Build history of the part. All positions in model axes, mm. Face numbers are marked on the shaded views. A direction names the side the tool comes from. Coordinates: 2 decimals unless noted, no trailing zeros. Loops run counter-clockwise (first coordinate to the right, second up) from the corner with the lowest first, then second, coordinate; pieces in that order, holes last.
Item 1: Drill centre lines: line 1 along Y through (x, z) = (5.5, 9.5); line 2 along Y through (x, z) = (112, 6); line 3 along X through (y, z) = (26, 7). Where is each one in solid material? Low to high.
Item 2: 3-axis set-ups, long thin cutter, end or side, ignore diameter. For the marked faces 5, 6 and 7: which of +Z, -Z, +X, -X, +Y, -Y reach the whole face in a straight line?
Item 3: Cut at B-B (x = 100). List the corners of the cut face in (y, z), and give its area (3 significant figures).
Item 4: Mould opens along X. For the marked faces 1, 2, 3 and 4 say: released by +X, released by -X, zero draft, split by the parting line, or undercut.
Item 5: Flat gauge pins, fed straight in: pin 1 (12 mm diameter, centred on x = 57, y = 47.5, fed in from +Z); pin 2 (2.5 mm diameter, centred on x = 104.5, z = 11, fed in from -Y); pin 3 (1.2 mm diameter, centred on x = 65.5, z = -7.5, fed in from +Y). Where does each tip first touch, or does it go through?
Item 6: Cut at C-C (z = -25). List the corners of the cut face in (x, y), and give its area (3 significant figures).
Item 7: Cut at D-D (x = 26). List the corners of the cut face in (y, z), and give its area (3 significant figures).
Item 8: Cut at A-A (y = 42.4). List the corners of the cut face in (x, z).
from build123d import *

# Parameters (mm, degrees)
SKETCH1_W               = 120
SKETCH1_H               = 45.4
BOSS_EXTRUDE1_DEPTH     = 12.5
SKETCH2_W               = 5
SKETCH2_H               = 45.4
BOSS_EXTRUDE2_DEPTH     = 10
CUT_EXTRUDE1_DEPTH      = 7.5
CUT_EXTRUDE1_DEPTH_BACK = 129.908533465
SKETCH3_W               = 78
SKETCH3_H               = 12.2
BOSS_EXTRUDE3_START     = -12.5
SKETCH4_W               = 42
SKETCH4_H               = 41
BOSS_EXTRUDE3_DEPTH     = 12.5
SKETCH5_R               = 15
SKETCH5_R_2             = 1.7
CUT_EXTRUDE2_DEPTH      = 138.38722648
SKETCH7_W               = 30
SKETCH7_H               = 8
BOSS_EXTRUDE4_DEPTH     = 44.5
SKETCH8_R               = 1.65
CUT_EXTRUDE4_DEPTH      = 148.030609058
FILLET1_SIZE            = 15
FILLET1_SIZE_2          = 6
SKETCH9_R               = 2.599999999
SKETCH9_R_2             = 12.000000007
CUT_EXTRUDE5_DEPTH      = 10
SKETCH10_R              = 3.5
CUT_EXTRUDE6_DEPTH      = 10.5
SKETCH12_R              = 3.5
CUT_EXTRUDE7_DEPTH      = 7.5
SKETCH6_W               = 105.644224039
SKETCH6_H               = 30.4
CUT_EXTRUDE3_DEPTH      = 10.5
CHAMFER1_SIZE           = 5
CHAMFER1_SIZE2          = 13.737387097
SKETCH13_W              = 14
SKETCH13_H              = 32.158687744
CUT_EXTRUDE8_DEPTH      = 10
SKETCH16_W              = 22.5
SKETCH16_H              = 11
CUT_EXTRUDE9_DEPTH      = 2
SKETCH18_W              = 3
SKETCH18_H              = 10.169703164
BOSS_EXTRUDE7_DEPTH     = 9.5
CUT_EXTRUDE10_REACH     = 144.298
SKETCH19_W              = 1.5
SKETCH19_H              = 14
SKETCH20_W              = 20
SKETCH20_H              = 5
CUT_EXTRUDE11_DEPTH     = 11
SKETCH21_R              = 1.5
CUT_EXTRUDE12_DEPTH     = 7
CHAMFER3_SIZE           = 1.5
FILLET3_R               = 5
CUT_EXTRUDE16_REACH     = 144.298
SKETCH24_W              = 5
SKETCH24_H              = 9
BOSS_EXTRUDE8_DEPTH     = 12.2
FILLET4_R               = 1
SKETCH15_R              = 2.75
BOSS_EXTRUDE9_DEPTH     = 2
CHAMFER4_SIZE           = 2
CHAMFER5_DEPTH          = 8


with BuildPart() as part:
    # Sketch1 → Boss-Extrude1 (new body)
    with BuildSketch(Plane.XY):
        with Locations((60, 22.7)):
            Rectangle(SKETCH1_W, SKETCH1_H)
    extrude(amount=BOSS_EXTRUDE1_DEPTH)

    # Sketch2 → Boss-Extrude2 (add)
    with BuildSketch(Plane(origin=(0, 0, 0), x_dir=(-1, 0, 0), z_dir=(0, 0, -1))):
        with Locations((-117.5, 22.7)):
            Rectangle(SKETCH2_W, SKETCH2_H)
    extrude(amount=BOSS_EXTRUDE2_DEPTH)

    # Sketch3 → Cut-Extrude1 (cut, two sides: drawn at the far end of the back side and taken through both)
    with BuildSketch(Plane.XY.offset(-CUT_EXTRUDE1_DEPTH_BACK)):
        with Locations((81, 22.8)):
            Rectangle(SKETCH3_W, SKETCH3_H)
    extrude(amount=CUT_EXTRUDE1_DEPTH + CUT_EXTRUDE1_DEPTH_BACK, mode=Mode.SUBTRACT)

    # Sketch4 → Boss-Extrude3 (add)
    with BuildSketch(Plane(origin=(0, 0, 0), x_dir=(-1, 0, 0), z_dir=(0, 0, -1)).offset(BOSS_EXTRUDE3_START)):
        with Locations((-21, 42.5)):
            Rectangle(SKETCH4_W, SKETCH4_H)
    extrude(amount=BOSS_EXTRUDE3_DEPTH)

    # Sketch5 → Cut-Extrude2 (cut, through all)
    with BuildSketch(Plane.XY.offset(12.5)):
        with Locations((21, 42.4)):
            Circle(SKETCH5_R)
        with Locations((5.5, 57.9)):
            Circle(SKETCH5_R_2)
        with Locations((36.5, 57.9)):
            Circle(SKETCH5_R_2)
        with Locations((36.5, 26.9)):
            Circle(SKETCH5_R_2)
        with Locations((5.5, 26.9)):
            Circle(SKETCH5_R_2)
    extrude(amount=-CUT_EXTRUDE2_DEPTH, mode=Mode.SUBTRACT)

    # Sketch7 → Boss-Extrude4 (add)
    with BuildSketch(Plane(origin=(0, 0, 0), x_dir=(-1, 0, 0), z_dir=(0, 0, -1))):
        with Locations((-65.5, 4)):
            Rectangle(SKETCH7_W, SKETCH7_H)
    extrude(amount=BOSS_EXTRUDE4_DEPTH)

    # Sketch8 → Cut-Extrude4 (cut, through all)
    with BuildSketch(Plane.XY.offset(12.5)):
        with Locations((91.5, 32.7)):
            Circle(SKETCH8_R)
        with Locations((111.5, 32.7)):
            Circle(SKETCH8_R)
        with Locations((111.5, 12.7)):
            Circle(SKETCH8_R)
        with Locations((91.5, 12.7)):
            Circle(SKETCH8_R)
    extrude(amount=-CUT_EXTRUDE4_DEPTH, mode=Mode.SUBTRACT)

    # Fillet1
    # a fillet whose section is not a circle: 15, 6 mm, written as the material it takes off along each edge
    with BuildSketch(Plane(origin=(50.5, -37.5, -44.5), x_dir=(1, 0, 0), z_dir=(0, 1, 0))) as fillet1_piece_1:
        with BuildLine():
            Bezier((FILLET1_SIZE, 0), (0, 0), (0, -FILLET1_SIZE_2), weights=[1, 0.428571429, 1])
            Line((0, -FILLET1_SIZE_2), (0, 0))
            Line((0, 0), (FILLET1_SIZE, 0))
        make_face()
    extrude(amount=83, mode=Mode.SUBTRACT)
    with BuildSketch(Plane(origin=(80.5, 45.5, -44.5), x_dir=(0, 0, 1), z_dir=(0, -1, 0))) as fillet1_piece_2:
        with BuildLine():
            Bezier((FILLET1_SIZE_2, 0), (0, 0), (0, FILLET1_SIZE), weights=[1, 0.428571429, 1])
            Line((0, FILLET1_SIZE), (0, 0))
            Line((0, 0), (FILLET1_SIZE_2, 0))
        make_face()
    extrude(amount=83, mode=Mode.SUBTRACT)

    # Sketch9 → Cut-Extrude5 (cut)
    with BuildSketch(Plane(origin=(0, 8, 0), x_dir=(1, 0, 0), z_dir=(0, 1, 0))):
        with Locations(Location((54.15539193, 34.815048574, 0), (0, 0, 180))):
            Circle(SKETCH9_R)
        with Locations(Location((65.469100429, 39.501340075, 0), (0, 0, 180))):
            Circle(SKETCH9_R)
        with Locations(Location((76.782808928, 34.815048574, 0), (0, 0, 180))):
            Circle(SKETCH9_R)
        with Locations(Location((65.469100429, 23.501340075, 0), (0, 0, 180))):
            Circle(SKETCH9_R_2)
    extrude(amount=-CUT_EXTRUDE5_DEPTH, mode=Mode.SUBTRACT)

    # Sketch10 → Cut-Extrude6 (cut)
    with BuildSketch(Plane.XY.offset(12.5)):
        with Locations((91.5, 32.7)):
            Circle(SKETCH10_R)
        with Locations((111.5, 32.7)):
            Circle(SKETCH10_R)
        with Locations((111.5, 12.7)):
            Circle(SKETCH10_R)
        with Locations((91.5, 12.7)):
            Circle(SKETCH10_R)
    extrude(amount=-CUT_EXTRUDE6_DEPTH, mode=Mode.SUBTRACT)

    # Sketch12 → Cut-Extrude7 (cut)
    with BuildSketch(Plane.XY.offset(12.5)):
        with Locations((36.5, 57.9)):
            Circle(SKETCH12_R)
        with Locations((5.5, 57.9)):
            Circle(SKETCH12_R)
        with Locations((5.5, 26.9)):
            Circle(SKETCH12_R)
        with Locations((36.5, 26.9)):
            Circle(SKETCH12_R)
    extrude(amount=-CUT_EXTRUDE7_DEPTH, mode=Mode.SUBTRACT)

    # Sketch6 → Cut-Extrude3 (cut)
    with BuildSketch(Plane.XY.offset(12.5)):
        with Locations((73.822112019, 47.8)):
            Rectangle(SKETCH6_W, SKETCH6_H)
    extrude(amount=-CUT_EXTRUDE3_DEPTH, mode=Mode.SUBTRACT)

    # Chamfer1
    chamfer1_edges = [part.edges().sort_by_distance(p)[0] for p in [
        (80.5, 4, 0),
    ]]
    chamfer1_side = [part.faces().sort_by_distance(p)[0] for p in [
        (40.688741063, 22.8, 0),
    ]]
    chamfer(chamfer1_edges, length=CHAMFER1_SIZE, length2=CHAMFER1_SIZE2, reference=chamfer1_side[0])

    # Sketch13 → Cut-Extrude8 (cut)
    with BuildSketch(Plane(origin=(0, 8, 0), x_dir=(1, 0, 0), z_dir=(0, 1, 0))):
        with Locations((65.469100429, 39.501340075)):
            Rectangle(SKETCH13_W, SKETCH13_H)
    extrude(amount=-CUT_EXTRUDE8_DEPTH, mode=Mode.SUBTRACT)

    # Sketch16 → Cut-Extrude9 (cut)
    with BuildSketch(Plane(origin=(120, 0, 0), x_dir=(0, 0, -1), z_dir=(1, 0, 0))):
        with Locations((-1.25, 5.5)):
            Rectangle(SKETCH16_W, SKETCH16_H)
    extrude(amount=-CUT_EXTRUDE9_DEPTH, mode=Mode.SUBTRACT)

    # Sketch18 → Boss-Extrude7 (add)
    with BuildSketch(Plane(origin=(0, 0, -10), x_dir=(-1, 0, 0), z_dir=(0, 0, -1))):
        with Locations((-116.5, 5.084851582)):
            Rectangle(SKETCH18_W, SKETCH18_H)
    extrude(amount=BOSS_EXTRUDE7_DEPTH)

    # Cut-Extrude10: up to this face of the body (flat: up to its plane)
    cut_extrude10_end = Plane(part.part.faces().sort_by_distance((119, 11, 1.25))[0])
    # Sketch19 → Cut-Extrude10 (cut, up to the picked face)
    with BuildSketch(Plane.XZ, mode=Mode.PRIVATE) as cut_extrude10_sk1:
        with Locations((117.25, -7)):
            Rectangle(SKETCH19_W, SKETCH19_H)
    cut_extrude10_tool1 = split(extrude(cut_extrude10_sk1.sketch, amount=-CUT_EXTRUDE10_REACH, mode=Mode.PRIVATE), bisect_by=cut_extrude10_end, keep=Keep.BOTH, mode=Mode.PRIVATE)
    add(cut_extrude10_tool1.solids().sort_by(Axis((117.25, 0, -7), (0, 1, 0)))[0], mode=Mode.SUBTRACT)

    # Sketch20 → Cut-Extrude11 (cut)
    with BuildSketch(Plane.XZ):
        with Locations((108, 10)):
            Rectangle(SKETCH20_W, SKETCH20_H)
    extrude(amount=-CUT_EXTRUDE11_DEPTH, mode=Mode.SUBTRACT)

    # Sketch21 → Cut-Extrude12 (cut)
    with BuildSketch(Plane(origin=(118, 0, 0), x_dir=(0, 0, -1), z_dir=(1, 0, 0))):
        with Locations((-2.485, 5)):
            Circle(SKETCH21_R)
        with Locations((16.565, 5)):
            Circle(SKETCH21_R)
    extrude(amount=-CUT_EXTRUDE12_DEPTH, mode=Mode.SUBTRACT)

    # Chamfer3
    chamfer3_edges = [part.edges().sort_by_distance(p)[0] for p in [
        (116.5, 5.084851582, -14),
        (116.5, 5.5, 0),
    ]]
    chamfer(chamfer3_edges, length=CHAMFER3_SIZE - 0.0001)  # a hair under: the kernel refuses the full size

    # Fillet3
    fillet3_edges = [part.edges().sort_by_distance(p)[0] for p in [
        (98, 11, 10),
    ]]
    fillet(fillet3_edges, radius=FILLET3_R)

    # Cut-Extrude16: up to this face of the body (flat: up to its plane)
    cut_extrude16_end = Plane(part.part.faces().sort_by_distance((42, 22.8, 3.75))[0])
    # Sketch23 → Cut-Extrude16 (cut, up to the picked face)
    with BuildSketch(Plane(origin=(120, 0, 0), x_dir=(0, 0, -1), z_dir=(1, 0, 0)), mode=Mode.PRIVATE) as cut_extrude16_sk1:
        Polygon((-6.5, 28.9), (-7.5, 28.9), (-7.5, 29.3), align=None)
    cut_extrude16_tool1 = split(extrude(cut_extrude16_sk1.sketch, amount=-CUT_EXTRUDE16_REACH, mode=Mode.PRIVATE), bisect_by=cut_extrude16_end, keep=Keep.BOTH, mode=Mode.PRIVATE)
    # Sketch23 → Cut-Extrude16 (cut, up to the picked face)
    with BuildSketch(Plane(origin=(120, 0, 0), x_dir=(0, 0, -1), z_dir=(1, 0, 0)), mode=Mode.PRIVATE) as cut_extrude16_sk2:
        Polygon((-7.5, 16.7), (-7.5, 16.3), (-6.5, 16.7), align=None)
    cut_extrude16_tool2 = split(extrude(cut_extrude16_sk2.sketch, amount=-CUT_EXTRUDE16_REACH, mode=Mode.PRIVATE), bisect_by=cut_extrude16_end, keep=Keep.BOTH, mode=Mode.PRIVATE)
    add(cut_extrude16_tool1.solids().sort_by(Axis((120, 29.033333, 7.166667), (-1, 0, 0)))[0], mode=Mode.SUBTRACT)
    add(cut_extrude16_tool2.solids().sort_by(Axis((120, 16.566667, 7.166667), (-1, 0, 0)))[0], mode=Mode.SUBTRACT)

    # Sketch24 → Boss-Extrude8 (add)
    with BuildSketch(Plane(origin=(0, 16.7, 0), x_dir=(1, 0, 0), z_dir=(0, 1, 0))):
        with Locations((117.5, 5.5)):
            Rectangle(SKETCH24_W, SKETCH24_H)
    extrude(amount=BOSS_EXTRUDE8_DEPTH)

    # Fillet4
    fillet4_edges = [part.edges().sort_by_distance(p)[0] for p in [
        (117.5, 28.9, -1),
        (117.5, 16.7, -1),
    ]]
    fillet(fillet4_edges, radius=FILLET4_R)

    # Sketch15 → Boss-Extrude9 (add)
    with BuildSketch(Plane(origin=(0, 8, 0), x_dir=(1, 0, 0), z_dir=(0, 1, 0))):
        with Locations((65.469100428, 7.501340074)):
            Circle(SKETCH15_R)
    extrude(amount=BOSS_EXTRUDE9_DEPTH)

    # Chamfer4
    chamfer4_edges = [part.edges().sort_by_distance(p)[0] for p in [
        (62.719100428, 10, -7.501340074),
    ]]
    chamfer(chamfer4_edges, length=CHAMFER4_SIZE - 0.0001)  # a hair under: the kernel refuses the full size

    # Chamfer5: read off the stored shape, not the designer's step
    # Chamfer5 outline → Chamfer5 (add)
    with BuildSketch(Plane(origin=(0, 0, 0), x_dir=(1, 0, 0), z_dir=(0, 1, 0))):
        with BuildLine():
            add(Edge.make_bspline(
                [(50.541922163, 38.782180687), (50.5, 38.636096407), (50.5, 38.5)],
                knots=[0.948627317, 0.948627317, 0.948627317, 1, 1, 1], degree=2, weights=[0.944304536, 0.970644181, 1]))
            Line((50.541922163, 38.782180687), (0, 0))
            Line((0, 0), (50.5, 0))
            Line((50.5, 0), (50.5, 38.5))
        make_face()
    extrude(amount=CHAMFER5_DEPTH)


solid = part.part
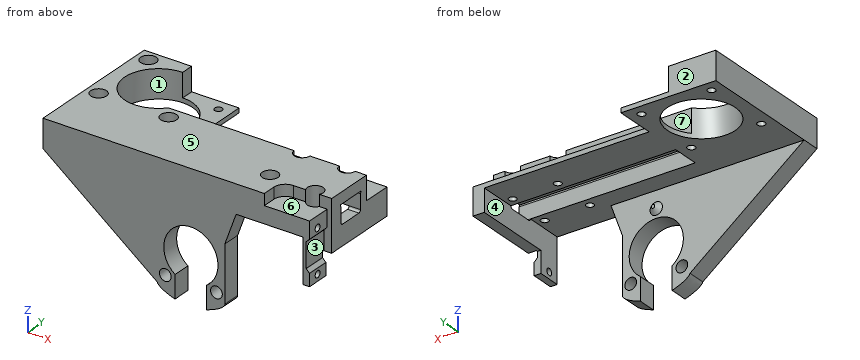
Filled sheet:
1. line 1: y = 0 to 23.4, 30.4 to 54.4, 61.4 to 63
1. line 2: y = 0 to 9.24, 16.16 to 16.7, 28.9 to 29.24
1. line 3: x = 0 to 2.12, 8.88 to 33.12, 39.88 to 42
2. face 5: +Z, +X, -X, +Y, -Y
2. face 6: +Z, +X, -Y
2. face 7: +Z, +X, +Y
3. outline: (0, 0) - (16.7, 0) - (16.7, 6.5) - (16.3, 7.5) - (29.3, 7.5) - (28.9, 6.5) - (28.9, 0) - (45.4, 0) - (45.4, 2) - (32.6, 2) - (32.6, 12.5) - (10, 12.5) - (10, 7.5) - (0, 7.5) - close
3. area: 291 mm2
4. face 1: undercut
4. face 2: zero draft
4. face 3: released by +X
4. face 4: undercut
5. pin 1: stops at z = 2
5. pin 2: stops at y = 11
5. pin 3: stops at y = 10
6. outline: (32.58, 0) - (53.56, 0) - (53.56, 8) - (32.58, 8) - close; (77.38, 0) - (80.5, 0) - (80.5, 8) - (77.38, 8) - close
6. area: 193 mm2
7. outline: (0, -19.95) - (8, -19.95) - (8, 0) - (28.26, 0) - (28.26, 12.5) - (0, 12.5) - close; (56.54, 0) - (63, 0) - (63, 2) - (56.54, 2) - close
7. area: 526 mm2
8. outline: (0, 0) - (6, 0) - (6, 12.5) - (0, 12.5) - close; (36, 0) - (115, 0) - (115, -10) - (120, -10) - (120, 2) - (36, 2) - close
